Geometry: see drawing. Coordinates: mm, zero at the bounding-box minimum. A direction names the side the tool comes from. Round coordinates to 2 decimals unless told otherwise and drop trailing zeros. Loops run counter-clockwise (first coordinate to the right, second up) from the corner with the lowest first, then second, coordinate; pieces in that order, holes last. Notation, with made-up numbers: (12.25, 52.25) - (22.25, 52.25) arc R15 cw to (22.25, 56.25) - close; hole circle Ø2 at (-16.5, -3.5). An arc over 180 degrees is marked (long way). Answer in a Markdown table with one row per item. Add a question column.
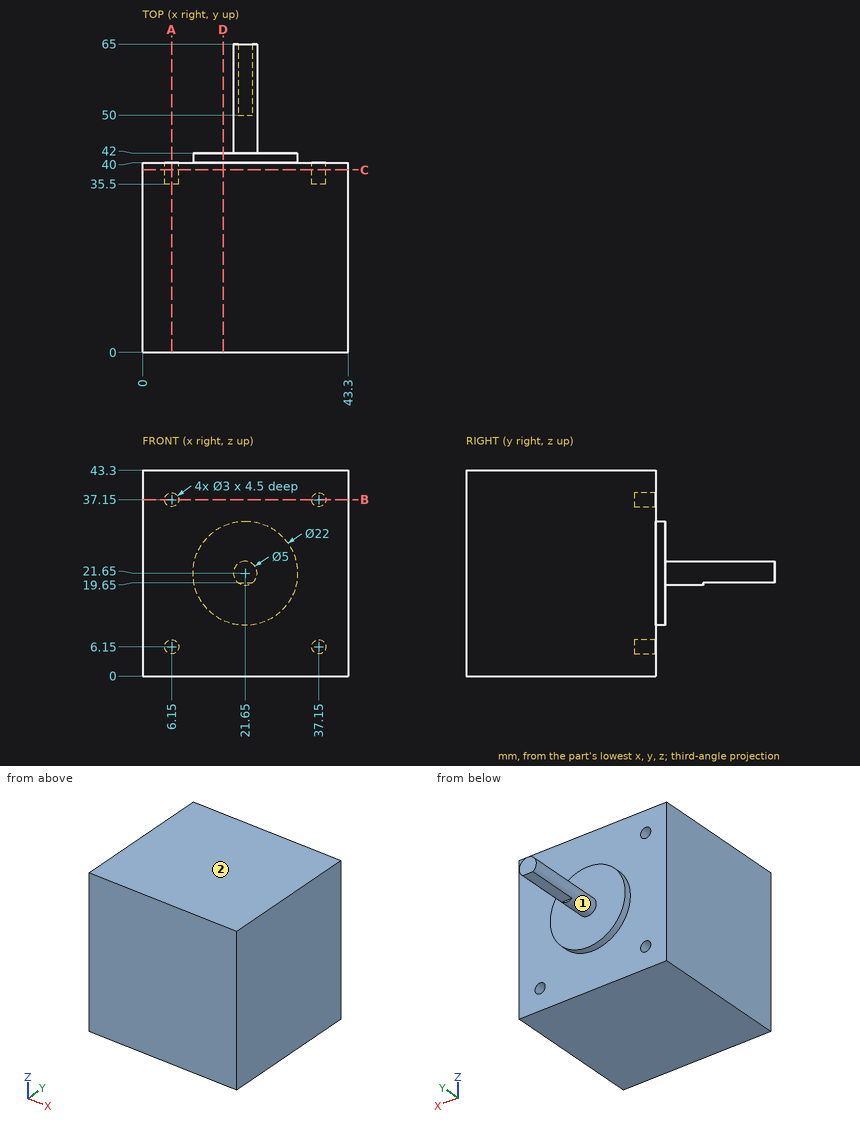
1) Section A-A, the plane x = 6.15. Return the cut outline in (y, z), and give its area (4 significant figures).
2) Section C-C, the plane y = 38.5. Return the cut outline in (x, z), and give its area (3 significant figures).
3) Contact query for flat-ended pins moving along their axis: pin 1 Ø3.5 at (x, z) = (37, 6) entering from +Y; pin 2 Ø5 at (x, z) = (6.15, 37.15) entering from -Y; pin 3 Ø3.5 at (x, y) = (21, 60.5) entering from -Z; pin 4 Ø8 at (x, z) = (32, 17.5) entering from +Y. Output: stop coordinate, or through.
4) Reachability of the marked faces 1 and 2 from +Z, -Z, +X, -X, +Y, -Y: full face, straight path, thin tool, end or side. Return the list, or none.
5) Section D-D, the plane x = 17. Return the cut outline in (y, z).
6) Section B-B, the plane z = 37.15. Return the cut outline in (x, y).
7) Material intervals for line 1 along X through (y, z) = (36, 37); line 2 along Y through (x, z) = (8, 6.5), sorted ascending. Write a range as from..to.
Evaluation:
| question | item | result |
|---|---|---|
| 1 | outline | (0, 0) - (40, 0) - (40, 4.65) - (35.5, 4.65) - (35.5, 7.65) - (40, 7.65) - (40, 35.65) - (35.5, 35.65) - (35.5, 38.65) - (40, 38.65) - (40, 43.3) - (0, 43.3) - close |
| 1 | area | 1,705 mm² |
| 2 | outline | (0, 0) - (43.3, 0) - (43.3, 43.3) - (0, 43.3) - close; hole circle Ø3 at (6.15, 6.15); hole circle Ø3 at (6.15, 37.15); hole circle Ø3 at (37.15, 6.15); hole circle Ø3 at (37.15, 37.15) |
| 2 | area | 1,850 mm² |
| 3 | pin 1 | stops at y = 40 |
| 3 | pin 2 | stops at y = 0 |
| 3 | pin 3 | stops at z = 19.65 |
| 3 | pin 4 | stops at y = 42 |
| 4 | face 1 | +Y |
| 4 | face 2 | +Z, +X, -X, +Y, -Y |
| 5 | outline | (0, 0) - (40, 0) - (40, 11.68) - (42, 11.68) - (42, 31.62) - (40, 31.62) - (40, 43.3) - (0, 43.3) - close |
| 6 | outline | (0, 0) - (43.3, 0) - (43.3, 40) - (38.65, 40) - (38.65, 35.5) - (35.65, 35.5) - (35.65, 40) - (7.65, 40) - (7.65, 35.5) - (4.65, 35.5) - (4.65, 40) - (0, 40) - close |
| 7 | line 1 | x = 0..4.66, 7.64..35.66, 38.64..43.3 |
| 7 | line 2 | y = 0..40 |
